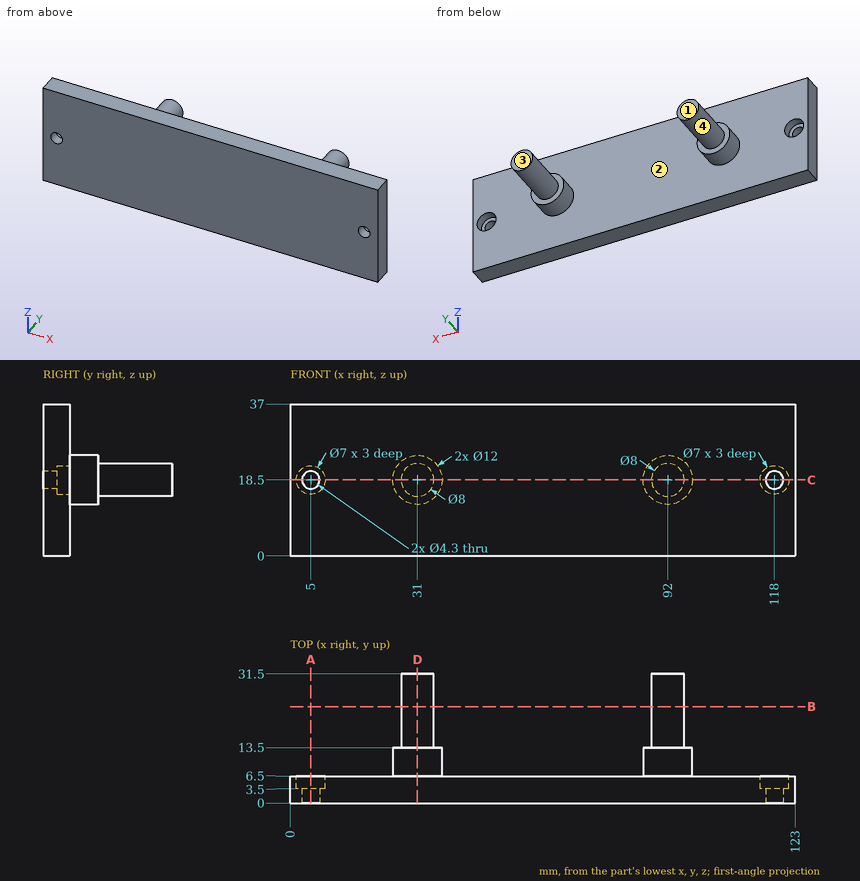
Geometry: see drawing. Coordinates: mm, zero at the bounding-box minimum. A direction names the side the tool comes from. Round coordinates to 2 decimals unless told otherwise and drop trailing zeros. Order: outer loops, then holes, each group sorted by start corner. A loop starts at its lowest first (then second) coordinate and runs counter-clockwise, first axis right, second up. Notation, with made-up numbers: (37.25, 11) -> (46.25, 11) arc R24 ccw to (46.25, 31) -> close; hole circle Ø1 at (17.5, 29.5). An arc over 180 degrees is marked (long way). Answer as CSV lines item,"result".
Item 1: Section D-D, the plane x = 31. Return loops of the section in (y, z).
A:
outline,"(0, 0) -> (6.5, 0) -> (6.5, 12.5) -> (13.5, 12.5) -> (13.5, 14.5) -> (31.5, 14.5) -> (31.5, 22.5) -> (13.5, 22.5) -> (13.5, 24.5) -> (6.5, 24.5) -> (6.5, 37) -> (0, 37) -> close"
Item 2: Reachability of the marked faces 3 and 4 from +Z, -Z, +X, -X, +Y, -Y: full face, straight path, thin tool, end or side. Return the list, or none.
A:
face 3,"+Z, -Z, +X, -X, +Y"
face 4,"+Y"
Item 3: Section C-C, the plane z = 18.5. Count the separate pieces of the cut face and the enclosed holes in it, plus the area to 3 significant figures.
A:
separate pieces,"3"
enclosed holes,"0"
area,"1,180 mm²"
Item 4: Pull-direction query (X, two-part tool) for the marked faces 1 and 2; classes: pulls with the +X half, pulls with the -X half, needs draft (parallel to the pull), parting line crosses it, or undercut.
A:
face 1,"needs draft"
face 2,"undercut"
Item 5: Pin query (flat end, axial travel): pin 1 Ø2.5 at (x, z) = (118, 18.5) entering from -Y; pin 2 Ø5 at (y, z) = (5, 11) entering from -X; pin 3 Ø1 at (x, y) = (28, 19.5) entering from +Z; pin 4 Ø1 at (x, z) = (42.5, 27) entering from +Y. Return the tip coordinate at first contact, or that it passes through.
A:
pin 1,"through"
pin 2,"x = 0"
pin 3,"z = 21.62"
pin 4,"y = 6.5"
Item 6: Line query: L1, parallel to X at y = 1.5, z = 18.5; L2, parallel to X at y = 4.65, z = 18.5; L3, parallel to Z at x = 5, y = 1.85. Output: solid intervals per line, ascending.
A:
L1,"0 to 2.85, 7.15 to 115.85, 120.15 to 123"
L2,"0 to 1.5, 8.5 to 114.5, 121.5 to 123"
L3,"0 to 16.35, 20.65 to 37"
Item 7: Section A-A, the plane x = 5. Return loops of the section in (y, z).
A:
outline,"(0, 0) -> (6.5, 0) -> (6.5, 15) -> (3.5, 15) -> (3.5, 16.35) -> (0, 16.35) -> close; (0, 20.65) -> (3.5, 20.65) -> (3.5, 22) -> (6.5, 22) -> (6.5, 37) -> (0, 37) -> close"
Item 8: Section B-B, the plane y = 23.5. Return loops of the section in (x, z).
A:
outline,"circle Ø8 at (31, 18.5); circle Ø8 at (92, 18.5)"
